Input: part model. Units: mm. Frame: model coordinates. Coordinates: 2 decimals unless noted, no trailing zeros. Order: outer loops, then holes, each group sorted by start corner. A loop starts at its lowest first (then second) coordinate and runs counter-clockwise, first axis right, second up. Notation, with made-up numbers: (67.25, 75.5) - (108.25, 75.5) arc R9 cw to (108.25, 82.5) - close; hole circle Ø4 at (2.5, -22). An arc over 180 degrees is marked (long way). Answer as CSV lines item,"result". Start each with the question number.
Item 1: Section A-A (z = 106). Output: boundary loops of the cut face in (x, y).
Item 2: First-contact query: pin 1 (5 mm diameter, centred on x = 7, z = -4, fed in from -Y); pin 2 (5 mm diameter, centred on x = 6, z = 149, fed in from -Y); pin 3 (5 mm diameter, centred on x = 7, y = 145.5, fed in from -Z). Flat tips, straight axial feed; report the tip coordinate or a pass-through.
Item 3: Material intervals for line 1 along Z through (x, y) = (3.5, 127.5); line 2 along Z through (x, y) = (2.75, 143.5); line 3 along Y through (x, z) = (3.5, 81.5), sorted ascending.
Item 4: Section C-C (z = 30.5). Output: boundary loops of the cut face in (x, y).
Item 5: Section B-B (y = 133). Output: boundary loops of the cut face in (x, z).
Item 6: Section D-D (x = 6.5). State how many separate pieces and enclosed holes the cut face has, and give its area (3 significant figures).
from build123d import *

# Parameters (mm, degrees)
SKETCH_W     = 10
SKETCH_H     = 40
SKETCH_H_2   = 29.8
PAD_DEPTH    = 10
SKETCH001_R  = 1.5
POCKET_DEPTH = 10.001


with BuildPart() as part:
    # Sketch → Pad (new body)
    with BuildSketch(Plane.YZ):
        Polygon((0, 0), (0, 22.5), (-10, 22.5), (-10, 92.5), (0, 92.5), (0, 152.5), (-10, 152.5), (-10, 222.5), (0, 222.5), (0, 250), (206.942136, 250), (223.276302, 233.665833), (216.205235, 226.594766), (237.277017, 205.522983), (244.348084, 212.594051), (265.561288, 191.380848), (258.49022, 184.30978), (279.562002, 163.237998), (286.63307, 170.309066), (307.704852, 149.237284), (300.633784, 142.166216), (330, 112.8), (320, 112.8), (320, 92.5), (330, 92.5), (330, 22.5), (320, 22.5), (320, 0), (289.5, 0), (289.5, -10), (209.5, -10), (209.5, 0), (110.5, 0), (110.5, -10), (30.5, -10), (30.5, 0), align=None)
        with Locations((35, 95.5)):
            Rectangle(SKETCH_W, SKETCH_H, mode=Mode.SUBTRACT)
        with Locations((146, 84.9)):
            Rectangle(SKETCH_W, SKETCH_H_2, mode=Mode.SUBTRACT)
        with Locations((146, 30.1)):
            Rectangle(SKETCH_W, SKETCH_H_2, mode=Mode.SUBTRACT)
        with Locations((174, 84.9)):
            Rectangle(SKETCH_W, SKETCH_H_2, mode=Mode.SUBTRACT)
        with Locations((174, 30.1)):
            Rectangle(SKETCH_W, SKETCH_H_2, mode=Mode.SUBTRACT)
        with BuildLine():
            Line((100, 175), (230, 175))
            ThreePointArc((240, 165), (237.071068, 172.071068), (230, 175))
            Line((240, 165), (240, 125))
            ThreePointArc((230, 115), (237.071068, 117.928932), (240, 125))
            Line((230, 115), (100, 115))
            ThreePointArc((90, 125), (92.928932, 117.928932), (100, 115))
            Line((90, 125), (90, 165))
            ThreePointArc((100, 175), (92.928932, 172.071068), (90, 165))
        make_face(mode=Mode.SUBTRACT)
        with BuildLine():
            ThreePointArc((189.86767, 232.075534), (182.796602, 232.075534), (182.796602, 225.004466))
            Line((182.796602, 225.004466), (189.86767, 217.933398))
            ThreePointArc((189.86767, 217.933398), (196.938737, 217.933398), (196.938737, 225.004466))
            Line((189.86767, 232.075534), (196.938737, 225.004466))
        make_face(mode=Mode.SUBTRACT)
        with BuildLine():
            ThreePointArc((210, 37.5), (202.5, 30), (210, 22.5))
            Line((210, 22.5), (250, 22.5))
            ThreePointArc((250, 22.5), (257.5, 30), (250, 37.5))
            Line((210, 37.5), (250, 37.5))
        make_face(mode=Mode.SUBTRACT)
    extrude(amount=PAD_DEPTH)

    # Sketch001 → Pocket (cut, through all)
    with BuildSketch(Plane.YZ):
        with Locations((72.5, 192)):
            Circle(SKETCH001_R)
        with Locations((86.5, 180.8)):
            Circle(SKETCH001_R)
        with Locations((113.5, 192)):
            Circle(SKETCH001_R)
        with Locations((127.5, 180.8)):
            Circle(SKETCH001_R)
    extrude(amount=POCKET_DEPTH, mode=Mode.SUBTRACT)


solid = part.part
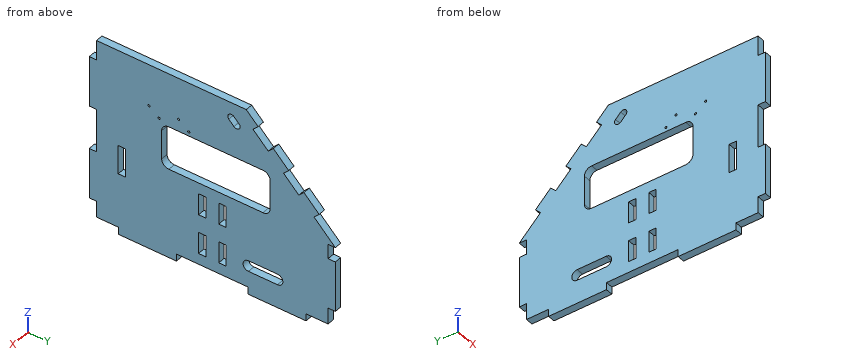
Determined:
1,outline,"(0, 0) - (10, 0) - (10, 30) - (0, 30) - close; (0, 40) - (10, 40) - (10, 320) - (0, 320) - close"
2,pin 1,"stops at y = 30.5"
2,pin 2,"stops at y = 0"
2,pin 3,"stops at z = 0"
3,line 1,"z = 0 to 115, 175 to 179.3, 182.3 to 250"
3,line 2,"z = 0 to 15.2, 45 to 70, 99.8 to 115, 175 to 250"
3,line 3,"y = -10 to 30, 40 to 141, 151 to 169, 179 to 330"
4,outline,"(0, -10) - (10, -10) - (10, 141) - (0, 141) - close; (0, 151) - (10, 151) - (10, 169) - (0, 169) - close; (0, 179) - (10, 179) - (10, 202.52) - (0, 202.52) - close; (0, 257.48) - (10, 257.48) - (10, 330) - (0, 330) - close"
5,outline,"(0, 0) - (10, 0) - (10, 115) - (0, 115) - close; (0, 175) - (10, 175) - (10, 250) - (0, 250) - close"
6,separate pieces,"1"
6,enclosed holes,"12"
6,area,"65,000 mm^2"
